Read the model definition and answer for the solid it produces. Units are mm, in the model's axes. A direction names the side the tool comes from. Give positions to 0.01 mm unless a question says otherwise; leave off trailing zeros. Loops run counter-clockwise (first coordinate to the right, second up) from the corner with the lowest first, then second, coordinate; pieces in that order, holes last. Notation, with made-up numbers: (29, 9.25) - (52, 9.25) arc R23 cw to (52, 24.25) - close; hole circle Ø2 at (-1, -7.5). An arc over 180 degrees is marked (long way). Use a Markdown table: item, result. Add a question column.
Item 1: A cutting plane is placed at B-B (z = -4). Determine the outline of the cut face in (x, y).
Item 2: Consider probe 1 along Y at (x, z) = (-279.4, -18.25); probe 2 along Y at (x, z) = (-523, -5.25); probe 3 along Z at (x, y) = (-274, 11). Determine where each line is inside the solid, lowest interval first. Write a range as [from, to].
Item 3: Which of the six approach directions +Z, -Z, +X, -X, +Y, -Y give full straight-line access (tool end or side, diameter ignored) to faces 1 (the face through (-275, 0, -9)), 2 (the face through (0, -1, -14))?
Item 4: Each of these flat-tipped pins is pushed along its axis until it touches: P1, Ø3, axis at x = -473, y = 7.5, coming from the +Z side; P2, Ø1.5, axis at x = -249, z = -12, coming from the +Y side. Where does it stop, or does it pass through?
Item 5: A cutting plane is placed at A-A (x = -238). Determine the outline of the cut face in (y, z), plus the area to 3 significant figures.
from build123d import *

# Parameters (mm, degrees)
F1_DEPTH = 558.8
F2_R     = 2.6162
F4_DEPTH = 25.4
F3_R     = 2.6162
F5_DEPTH = 25.4


with BuildPart() as f1:
    # F0 (on Right) → F1 (new body)
    with BuildSketch(Plane.YZ):
        Polygon((0, -17.4625), (0, 0), (-1.5875, 0), (-1.5875, -19.05), (17.4625, -19.05), (17.4625, -17.4625), align=None)
    extrude(amount=-F1_DEPTH)

    # F2 (on face) → F4 (cut)
    with BuildSketch(Plane(origin=(0, 0, 0), x_dir=(-1, 0, 0), z_dir=(0, 1, 0))):
        with Locations((7.1501, -10.3251)):
            Circle(F2_R)
        with Locations((551.6499, -10.3251)):
            Circle(F2_R)
    extrude(amount=-F4_DEPTH, mode=Mode.SUBTRACT)

    # F3 (on face) → F5 (cut)
    with BuildSketch(Plane.XY.offset(-17.4625)):
        with Locations((-8.73125, 8.73125)):
            Circle(F3_R)
        with Locations((-550.06875, 8.73125)):
            Circle(F3_R)
        with Locations((-50.8, 8.73125)):
            Circle(F3_R)
        with Locations((-127, 8.73125)):
            Circle(F3_R)
        with Locations((-203.2, 8.73125)):
            Circle(F3_R)
        with Locations((-279.4, 8.73125)):
            Circle(F3_R)
        with Locations((-355.6, 8.73125)):
            Circle(F3_R)
        with Locations((-431.8, 8.73125)):
            Circle(F3_R)
        with Locations((-508, 8.73125)):
            Circle(F3_R)
    extrude(amount=-F5_DEPTH, mode=Mode.SUBTRACT)


solid = f1.part
Geometry says:
| question | item | result |
|---|---|---|
| 1 | outline | (-558.8, -1.59) - (0, -1.59) - (0, 0) - (-558.8, 0) - close |
| 2 | probe 1 | [-1.59, 6.12], [11.35, 17.46] |
| 2 | probe 2 | [-1.59, 0] |
| 2 | probe 3 | [-19.05, -17.46] |
| 3 | face 1 | +Z, +X, -X, +Y |
| 3 | face 2 | +Z, -Z, +X, +Y, -Y |
| 4 | P1 | z = -17.46 |
| 4 | P2 | y = 0 |
| 5 | outline | (-1.59, -19.05) - (17.46, -19.05) - (17.46, -17.46) - (0, -17.46) - (0, 0) - (-1.59, 0) - close |
| 5 | area | 58.0 mm² |
